from build123d import *

# Parameters (mm, degrees)
SKETCH1_R           = 8
SKETCH1_R_2         = 5
BOSS_EXTRUDE1_DEPTH = 20
SKETCH2_R           = 5
CUT_EXTRUDE1_DEPTH  = 35


with BuildPart() as part:
    # Sketch1 → Boss-Extrude1 (new body)
    with BuildSketch(Plane.XY):
        with BuildLine():
            Line((-10, 0), (-150, 0))
            ThreePointArc((-150, 0), (-175, -25), (-150, -50))
            Line((-150, -50), (-38.867513459, -50))
            ThreePointArc((-38.867513459, -50), (-31.796445648, -52.928932188), (-28.867513459, -60))
            Line((-28.867513459, -60), (-28.867513459, -100))
            ThreePointArc((-28.867513459, -100), (-14.43375673, -114.43375673), (0, -100))
            Line((0, -100), (0, -10))
            ThreePointArc((0, -10), (-2.928932188, -2.928932188), (-10, 0))
        make_face()
        with Locations((-150, -25)):
            Circle(SKETCH1_R, mode=Mode.SUBTRACT)
        with Locations((-14.43375673, -100)):
            Circle(SKETCH1_R_2, mode=Mode.SUBTRACT)
    extrude(amount=BOSS_EXTRUDE1_DEPTH)

    # Sketch2 → Cut-Extrude1 (cut)
    with BuildSketch(Plane.XY.offset(20)):
        with Locations((-45, -26.406771576)):
            Circle(SKETCH2_R)
    extrude(amount=-CUT_EXTRUDE1_DEPTH, mode=Mode.SUBTRACT)


solid = part.part
Could you check a few things on this model? Use its own coordinates, in mm. A direction names the side the tool comes from. Coordinates: 2 decimals unless noted, no trailing zeros. Order: outer loops, then holes, each group sorted by start corner. A loop starts at its lowest first (then second) coordinate and runs counter-clockwise, first axis right, second up. Notation, with made-up numbers: (35, -12) - (44, -12) arc R23 cw to (44, 6) - close; hole circle Ø1 at (-25.5, -18.75). An arc over 180 degrees is marked (long way). Answer in a Markdown table with one row per item. Add a question column.
(1) If we mould it in two halves opening along Y, with no side actions, what happens to faces 1 (the face through (-48.968, -29.449, 10.14)), 2 (the face through (0, -56, 10)), 3 (the face through (-14.75, -114.43, 9.86))? For each: released by +Y, released by -Y, zero draft, split by the parting line, or undercut.
(2) If we section it at A-A, the plane z = 15.75: Please give me the cut outline in (x, y), then the cut area to 3 significant figures.
(3) If we section it at C-C, the plane y = -67: Please give me the cut outline in (x, z).
(4) On a 3-axis mill with a long thin cutter (end or side, diameter ignored), from which of +Z, -Z, +X, -X, +Y, -Y can I reach the whole of each face in a straight line? I mean faces 4 (the face through (-28.868, -80, 10)), 5 (the face through (-2.85, -3.01, 9.86)). Say none if no direction works.
(5) Will these pins go through, and if not, where does the flat tip stop? pin 1 (1.5 mm diameter, centred on x = -152.5, z = 17, fed in from -Y); pin 2 (8 mm diameter, centred on x = -41, z = 10.5, fed in from -Y); pin 3 (12 mm diameter, centred on y = -24.5, z = 10, fed in from -X).
(6) I need wall thicknesses on L1, parallel to X at y = -28, z = 6.5; L2, parallel to Y at x = -150, z = 14.75; L3, parallel to Y at x = -45, z = 4.25. Which ranges of each line are inside material? Lowest first, please.
(7) If we section it at B-B, the plane x = -86.5: Please give me the cut outline in (y, z).
Results are:
| question | item | result |
|---|---|---|
| 1 | face 1 | undercut |
| 1 | face 2 | zero draft |
| 1 | face 3 | released by -Y |
| 2 | outline | (-150, -50) - (-38.87, -50) arc R10 cw to (-28.87, -60) - (-28.87, -100) arc R14.43 ccw to (0, -100) - (0, -10) arc R10 ccw to (-10, 0) - (-150, 0) arc R25 ccw to start; hole circle Ø16 at (-150, -25); hole circle Ø10 at (-45, -26.41); hole circle Ø10 at (-14.43, -100) |
| 2 | area | 9,890 mm2 |
| 3 | outline | (-28.87, 0) - (0, 0) - (0, 20) - (-28.87, 20) - close |
| 4 | face 4 | +Z, -Z, -X, -Y |
| 4 | face 5 | +Z, -Z, +X, +Y |
| 5 | pin 1 | stops at y = -49.94 |
| 5 | pin 2 | stops at y = -50.18 |
| 5 | pin 3 | stops at x = -175 |
| 6 | L1 | x = -174.82 to -157.42, -142.58 to -49.74, -40.26 to 0 |
| 6 | L2 | y = -50 to -33, -17 to 0 |
| 6 | L3 | y = -50 to -31.41, -21.41 to 0 |
| 7 | outline | (-50, 0) - (0, 0) - (0, 20) - (-50, 20) - close |
